from build123d import *

# Parameters (mm, degrees)
SKETCH2_W            = 40.2336
SKETCH2_H            = 25.019
SKETCH2_R            = 1.05
BOSS_EXTRUDE1_DEPTH  = 1.5
BOSS_EXTRUDE2_DEPTH  = 6.35
SKETCH4_R            = 8
BOSS_EXTRUDE3_DEPTH  = 9.2
SKETCH5_R            = 5.95
BOSS_EXTRUDE4_DEPTH  = 2.36
SKETCH6_R            = 7
BOSS_EXTRUDE5_DEPTH  = 4
SKETCH7_W            = 4.22
SKETCH7_H            = 7.75
BOSS_EXTRUDE6_DEPTH  = 8.3
SKETCH8_W            = 9
SKETCH8_H            = 2.93
BOSS_EXTRUDE7_DEPTH  = 4.35
SKETCH9_W            = 3.1
SKETCH9_H            = 5
BOSS_EXTRUDE8_DEPTH  = 1.3
SKETCH10_W           = 25.5
SKETCH10_H           = 8
BOSS_EXTRUDE9_DEPTH  = 1.4
SKETCH11_W           = 1.3
SKETCH11_H           = 2
BOSS_EXTRUDE10_DEPTH = 1.6
SKETCH12_W           = 3
SKETCH12_H           = 3
BOSS_EXTRUDE11_DEPTH = 1.4


with BuildPart() as part:
    # Sketch2 → Boss-Extrude1 (new body)
    with BuildSketch(Plane.XY):
        Rectangle(SKETCH2_W, SKETCH2_H)
        with Locations((-18.4568, 10.8495)):
            Circle(SKETCH2_R, mode=Mode.SUBTRACT)
        with Locations(Location((-18.4568, -10.8495, 0), (0, 0, 180))):
            Circle(SKETCH2_R, mode=Mode.SUBTRACT)
        with Locations((18.4568, -10.8495)):
            Circle(SKETCH2_R, mode=Mode.SUBTRACT)
        with Locations(Location((18.4568, 10.8495, 0), (0, 0, 180))):
            Circle(SKETCH2_R, mode=Mode.SUBTRACT)
    extrude(amount=BOSS_EXTRUDE1_DEPTH)

    # Sketch3 → Boss-Extrude2 (add)
    with BuildSketch(Plane.XY.offset(1.5)):
        with BuildLine():
            Line((-8.4, -2.05), (-8.4, -8.4))
            Line((-8.4, -8.4), (8.4, -8.4))
            Line((8.4, -8.4), (8.4, -2.05))
            Line((8.4, -2.05), (10.7, -2.05))
            ThreePointArc((10.7, -2.05), (12.75, 0), (10.7, 2.05))
            Line((10.7, 2.05), (8.4, 2.05))
            Line((8.4, 2.05), (8.4, 8.4))
            Line((8.4, 8.4), (-8.4, 8.4))
            Line((-8.4, 8.4), (-8.4, 2.05))
            Line((-8.4, 2.05), (-10.7, 2.05))
            ThreePointArc((-10.7, 2.05), (-12.75, 0), (-10.7, -2.05))
            Line((-10.7, -2.05), (-8.4, -2.05))
        make_face()
    extrude(amount=BOSS_EXTRUDE2_DEPTH)

    # Sketch4 → Boss-Extrude3 (add)
    with BuildSketch(Plane.XY.offset(7.85)):
        Circle(SKETCH4_R)
    extrude(amount=BOSS_EXTRUDE3_DEPTH)

    # Sketch5 → Boss-Extrude4 (add)
    with BuildSketch(Plane.XY.offset(17.05)):
        Circle(SKETCH5_R)
    extrude(amount=BOSS_EXTRUDE4_DEPTH)

    # Sketch6 → Boss-Extrude5 (add)
    with BuildSketch(Plane.XY.offset(19.41)):
        Circle(SKETCH6_R)
    extrude(amount=BOSS_EXTRUDE5_DEPTH)

    # Sketch7 → Boss-Extrude6 (add)
    with BuildSketch(Plane(origin=(0, 0, 0), x_dir=(-1, 0, 0), z_dir=(0, 0, -1))):
        with Locations((-17.5068, 0)):
            Rectangle(SKETCH7_W, SKETCH7_H)
    extrude(amount=BOSS_EXTRUDE6_DEPTH)

    # Sketch8 → Boss-Extrude7 (add)
    with BuildSketch(Plane(origin=(0, 0, 0), x_dir=(-1, 0, 0), z_dir=(0, 0, -1))):
        with Locations((11.1768, -9.4045)):
            Rectangle(SKETCH8_W, SKETCH8_H)
    extrude(amount=BOSS_EXTRUDE7_DEPTH)

    # Sketch9 → Boss-Extrude8 (add)
    with BuildSketch(Plane.XY.offset(1.5)):
        with Locations((13.0668, 8.5095)):
            Rectangle(SKETCH9_W, SKETCH9_H)
    extrude(amount=BOSS_EXTRUDE8_DEPTH)

    # Sketch10 → Boss-Extrude9 (add)
    with BuildSketch(Plane(origin=(0, 0, 0), x_dir=(-1, 0, 0), z_dir=(0, 0, -1))):
        with Locations((-0.3668, 8.2095)):
            Rectangle(SKETCH10_W, SKETCH10_H)
    extrude(amount=BOSS_EXTRUDE9_DEPTH)

    # Sketch11 → Boss-Extrude10 (add)
    with BuildSketch(Plane.XY.offset(1.5)):
        with Locations((14.7668, -9.5095)):
            Rectangle(SKETCH11_W, SKETCH11_H)
        with Locations((-17.777092667, 6.391636208)):
            Rectangle(SKETCH11_W, SKETCH11_H)
    extrude(amount=BOSS_EXTRUDE10_DEPTH)

    # Sketch12 → Boss-Extrude11 (add)
    with BuildSketch(Plane(origin=(0, 0, 0), x_dir=(-1, 0, 0), z_dir=(0, 0, -1))):
        with Locations((17.6168, 6.6095)):
            Rectangle(SKETCH12_W, SKETCH12_H)
    extrude(amount=BOSS_EXTRUDE11_DEPTH)


solid = part.part
Input: part model. Units: mm. Frame: model coordinates. A direction names the side the tool comes from. Coordinates: 2 decimals unless noted, no trailing zeros. Order: outer loops, then holes, each group sorted by start corner. A loop starts at its lowest first (then second) coordinate and runs counter-clockwise, first axis right, second up.
1. Cut plane C-C, the plane x = -14.5. Return loops of the section in (y, z), plus the area to 3 significant figures.
Checked values:
outline: (-12.51, 0) - (-10.87, 0) - (-10.87, -4.35) - (-7.94, -4.35) - (-7.94, 0) - (12.51, 0) - (12.51, 1.5) - (-12.51, 1.5) - close
area: 50.3 mm2
2. Access query for faces 1 (the flat face through (-11, -7.94, -2)), 2 (the flat face through (13, 6.009, 2)), 3 (the flat face through (13.117, 8, -1)), 4 (the flat face through (-18.427, 6, 2)), 5 (the flat face through (18, -3.875, -4)). Directions: +Z, -Z, +X, -X, +Y, -Y. A direction counts if a zero-diameter tool reaches every point of the face in a straight line with its end or side. Return the directions, or none.
Checked values:
face 1: -Z, +X, -X
face 2: +Z, +X
face 3: -Z, +X, +Y, -Y
face 4: +Z, -X, +Y, -Y
face 5: -Z, +X, -X, -Y
3. Cut plane A-A, the plane z = -0.5. Return loops of the section in (x, y) (1 decimal).
Checked values:
outline: (-19.1, 5.1) - (-16.1, 5.1) - (-16.1, 8.1) - (-19.1, 8.1) - close; (-15.7, -10.9) - (-6.7, -10.9) - (-6.7, -7.9) - (-15.7, -7.9) - close; (-12.4, 4.2) - (13.1, 4.2) - (13.1, 12.2) - (-12.4, 12.2) - close; (15.4, -3.9) - (19.6, -3.9) - (19.6, 3.9) - (15.4, 3.9) - close
4. Cut plane B-B, the plane y = 0. Return loops of the section in (x, z), plus the area to 3 significant figures.
Checked values:
outline: (-20.12, 0) - (15.4, 0) - (15.4, -8.3) - (19.62, -8.3) - (19.62, 0) - (20.12, 0) - (20.12, 1.5) - (12.75, 1.5) - (12.75, 7.85) - (8, 7.85) - (8, 17.05) - (5.95, 17.05) - (5.95, 19.41) - (7, 19.41) - (7, 23.41) - (-7, 23.41) - (-7, 19.41) - (-5.95, 19.41) - (-5.95, 17.05) - (-8, 17.05) - (-8, 7.85) - (-12.75, 7.85) - (-12.75, 1.5) - (-20.12, 1.5) - close
area: 489 mm2
5. Ray query, line 1 along Y through (x, z) = (-9.5, -1); line 2 along Z through (x, y) = (4.5, -4.25); line 3 along Z through (x, y) = (12.5, -4.25). Return the intervals inside material, ascending.
Checked values:
line 1: y = -10.87 to -7.94, 4.21 to 12.21
line 2: z = 0 to 17.05, 19.41 to 23.41
line 3: z = 0 to 1.5
6. Contact query for flat-ended pins moving along their axis: P1, Ø4, axis at y = -2.5, z = 8.5, coming from the -X side; P2, Ø3, axis at x = -2, z = -3, coming from the -Y side; P3, Ø0.7, axis at y = 7, z = -0.5, coming from the -X side; P4, Ø0.7, axis at x = 15, z = 2.5, coming from the -Y side. Output: stop coordinate, or through.
Checked values:
P1: stops at x = -12.66
P2: passes through
P3: stops at x = -19.12
P4: stops at y = -10.51
7. Cut plane D-D, the plane x = 9.5. Return loops of the section in (y, z), plus the area to 3 significant figures.
Checked values:
outline: (-12.51, 0) - (4.21, 0) - (4.21, -1.4) - (12.21, -1.4) - (12.21, 0) - (12.51, 0) - (12.51, 1.5) - (2.05, 1.5) - (2.05, 7.85) - (-2.05, 7.85) - (-2.05, 1.5) - (-12.51, 1.5) - close
area: 74.8 mm2
8. Draft query along X for faces 6 (the flat face through (8.4, -5, 5)), 7 (the flat face through (-20.117, 0, 1)), 8 (the flat face through (-12.383, 8, -1)). Return one class per face: +X half, -X half, draft (parallel to the pull), parting line (faces both ways), or undercut.
Checked values:
face 6: +X half
face 7: -X half
face 8: undercut
